CAD build for the part. Positions are in the model's coordinates, mm. Face numbers are marked on the shaded views. A direction names the side the tool comes from. Coordinates: 2 decimals unless noted, no trailing zeros. Loops run counter-clockwise (first coordinate to the right, second up) from the corner with the lowest first, then second, coordinate; pieces in that order, holes last.
1) Saw through at C-C, the plane z = 0. Write the cut outline in (x, y).
2) Two-plate mould, pull along X, no slides. Class the marked faces 3, 4, 5 and 6: +X half, -X half, draft (parallel to the pull), parting line (faces both ways), or undercut.
3) Saw through at B-B, the plane y = -4. Write the cut outline in (x, z).
4) Saw through at A-A, the plane x = 0. Write the cut outline in (y, z), and give its area (3 significant figures).
5) Which spindle directions (+Z, -Z, +X, -X, +Y, -Y) get a long thin tool onto all of the face, cutting with end or side? Do the marked faces 1 and 2. Say none if no direction does.
6) Pin check, flat tips, straight feed: pin 1 Ø2 at (x, y) = (0, -7) entering from -Z; pin 2 Ø4 at (x, y) = (3.5, 20) entering from -Z; pin 3 Ø1 at (y, z) = (38.5, -3.5) entering from +X; pin 4 Ø3 at (x, y) = (0, -4) entering from -Z. Stop position of each tip, or through.
7) Saw through at D-D, the plane x = 2.75. Write the cut outline in (y, z), and give its area (3 significant figures).
8) Wall check: line 1 along Y through (x, z) = (0, -0.3); line 2 along Y through (x, z) = (-0.75, -3.5); line 3 along X through (y, z) = (44.5, 2.5). Give the ranges that are in metal, low to high.
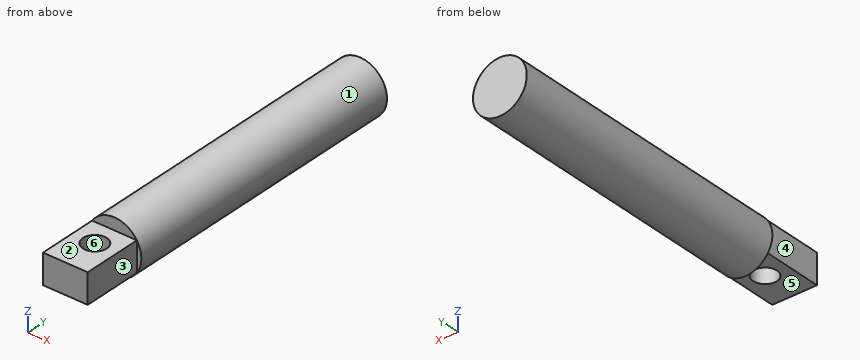
```python
from build123d import *

# Parameters (mm, degrees)
SKETCH1_R           = 4.5
BOSS_EXTRUDE1_DEPTH = 50
SKETCH2_W           = 7.48845263
SKETCH2_H           = 4.992301796
BOSS_EXTRUDE2_DEPTH = 10
SKETCH3_R           = 2
CUT_EXTRUDE1_DEPTH  = 10


with BuildPart() as part:
    # Sketch1 → Boss-Extrude1 (new body)
    with BuildSketch(Plane(origin=(0, 0, 0), x_dir=(1, 0, 0), z_dir=(0, 1, 0))):
        Circle(SKETCH1_R)
    extrude(amount=BOSS_EXTRUDE1_DEPTH)

    # Sketch2 → Boss-Extrude2 (add)
    with BuildSketch(Plane.XZ):
        Rectangle(SKETCH2_W, SKETCH2_H)
    extrude(amount=BOSS_EXTRUDE2_DEPTH)

    # Sketch3 → Cut-Extrude1 (cut)
    with BuildSketch(Plane(origin=(0, 0, -2.496150898), x_dir=(-1, 0, 0), z_dir=(0, 0, -1))):
        with Locations((0, -4)):
            Circle(SKETCH3_R)
    extrude(amount=-CUT_EXTRUDE1_DEPTH, mode=Mode.SUBTRACT)


solid = part.part
```
Data:
1. outline: (-4.5, 0) - (-3.74, 0) - (-3.74, -10) - (3.74, -10) - (3.74, 0) - (4.5, 0) - (4.5, 50) - (-4.5, 50) - close; hole circle Ø4 at (0, -4)
2. face 3: +X half
2. face 4: -X half
2. face 5: draft
2. face 6: undercut
3. outline: (-3.74, -2.5) - (-2, -2.5) - (-2, 2.5) - (-3.74, 2.5) - close; (2, -2.5) - (3.74, -2.5) - (3.74, 2.5) - (2, 2.5) - close
4. outline: (-10, -2.5) - (-6, -2.5) - (-6, 2.5) - (-10, 2.5) - close; (-2, -2.5) - (0, -2.5) - (0, -4.5) - (50, -4.5) - (50, 4.5) - (0, 4.5) - (0, 2.5) - (-2, 2.5) - close
4. area: 480 mm2
5. face 1: +Y, -Y
5. face 2: +Z, +X, -X, -Y
6. pin 1: stops at z = -2.5
6. pin 2: stops at z = -4.24
6. pin 3: stops at x = 3.35
6. pin 4: passes through
7. outline: (-10, -2.5) - (0, -2.5) - (0, -3.56) - (50, -3.56) - (50, 3.56) - (0, 3.56) - (0, 2.5) - (-10, 2.5) - close
7. area: 406 mm2
8. line 1: y = -10 to -6, -2 to 50
8. line 2: y = 0 to 50
8. line 3: x = -3.74 to 3.74
